For this review, take the finished solid that the model builds, in its own axes (mm). A direction names the side the tool comes from. Coordinates: 2 decimals unless noted, no trailing zeros. Loops run counter-clockwise (first coordinate to the right, second up) from the corner with the lowest first, then second, coordinate; pieces in that order, holes last.
1. Take a section at D-D, the plane z = -22. State the section outline as (x, y) points, then the cut area to 3 significant figures.
2. Machinability: for faces 1 (the face through (12.7, 8, 15)), 2 (the face through (6, -29, 11.659)), which of the approach directions +Z, -Z, +X, -X, +Y, -Y give a long, thin tool a straight path to every point of the face, cutting with its end or side? Answer none if there is none.
3. To check wall thickness, follow probe 1 along Y at (x, z) = (2.75, 17.5); probe 2 along Z at (x, y) = (5.25, -46); probe 3 along Y at (x, z) = (6, -41). State the ranges of each line that lie inside material, in increasing order.
4. Take a section at C-C, the plane y = -35. State the section outline as (x, z) points, then the cut area to 3 significant figures.
5. Mouldability with a two-part tool opening along Z and no side actions: class faces 3 (the face through (6.261, 37.248, -43.974)), 4 (the face through (6.261, -48.266, 16.077)), 5 (the face through (6, -29, 37.059)), 6 (the face through (6.261, -40.847, 33.857)) as pulls with the +Z half, pulls with the -Z half, needs draft (parallel to the pull), parting line crosses it, or undercut.
6. Clearance check with flat-ended pins moving along their axes: P1, Ø2, axis at x = 10.5, z = 0, coming from the -Y side; P2, Ø3, axis at x = 8.5, y = 29, coming from the +Z side; P3, Ø1.5, axis at x = 4.5, y = -36, coming from the -Z side. State where each tip first meets the part, or that it passes through.
7. Take a section at B-B, the plane z = 19.5. State the section outline as (x, y) points, then the cut area to 3 significant figures.
8. Take a section at A-A, the plane x = 4. State the section outline as (y, z) points (3 decimals).
```python
from build123d import *

# Parameters (mm, degrees)
F1_DEPTH = 12.7
F3_D     = 6.35


with BuildPart() as f1:
    # F0 (on Right) → F1 (new body)
    with BuildSketch(Plane.YZ):
        with BuildLine():
            Line((-57.135387, 37.059388), (-57.135387, 11.659388))
            Line((-57.135387, 11.659388), (-0.673995, 11.659388))
            ThreePointArc((-0.673995, 11.659388), (17.286517, 4.219901), (24.726005, -13.740612))
            Line((24.726005, -13.740612), (24.726005, -42.315612))
            Line((24.726005, -42.315612), (50.126005, -45.680172))
            Line((50.126005, -45.680172), (50.126005, -13.740612))
            ThreePointArc((50.126005, -13.740612), (35.247029, 22.180413), (-0.673995, 37.059388))
            Line((-0.673995, 37.059388), (-57.135387, 37.059388))
        make_face()
    extrude(amount=F1_DEPTH)

    # F3 (through all)
    with Locations(Plane.YZ.offset(12.7)):
        with Locations((-50.785387, 18.009388), (-41.260387, 30.709388)):
            Hole(F3_D / 2)


solid = f1.part
```
Results list:
1. outline: (0, 24.73) - (12.7, 24.73) - (12.7, 50.13) - (0, 50.13) - close
1. area: 323 mm2
2. face 1: +Z, -Z, +X, +Y, -Y
2. face 2: -Z, +X, -X, -Y
3. probe 1: y = -57.14 to -53.92, -47.65 to 39.38
3. probe 2: z = 11.66 to 37.06
3. probe 3: y = 24.73 to 50.13
4. outline: (0, 11.66) - (12.7, 11.66) - (12.7, 37.06) - (0, 37.06) - close
4. area: 323 mm2
5. face 3: pulls with the -Z half
5. face 4: undercut
5. face 5: pulls with the +Z half
5. face 6: undercut
6. P1: stops at y = 20.01
6. P2: stops at z = 28.53
6. P3: stops at z = 11.66
7. outline: (0, -57.14) - (12.7, -57.14) - (12.7, -53.59) - (0, -53.59) - close; (0, -47.98) - (12.7, -47.98) - (12.7, 37.74) - (0, 37.74) - close
7. area: 1,130 mm2
8. outline: (-57.135, 11.659) - (-0.674, 11.659) arc R25.4 cw to (24.726, -13.741) - (24.726, -42.316) - (50.126, -45.68) - (50.126, -13.741) arc R50.8 ccw to (-0.674, 37.059) - (-57.135, 37.059) - close; hole circle Ø6.35 at (-50.785, 18.009); hole circle Ø6.35 at (-41.26, 30.709)
